Verification items for the finished model (mm, model axes). A direction names the side the tool comes from. Coordinates: 2 decimals unless noted, no trailing zeros. Loops run counter-clockwise (first coordinate to the right, second up) from the corner with the lowest first, then second, coordinate; pieces in that order, holes last. Notation, with made-up numbers: (72.25, 19) -> (100.25, 19) arc R11 cw to (100.25, 31) -> close; hole circle Ø5 at (-35, 69.5). An arc over 180 degrees is marked (long way). Answer as a JSON object with one key per item and string values. Group by question number.
Q1. Release check for a two-part mould opening along Y. For faces 5 (the cylindrical face through (1467.341, 1019.425, 1.815)), 6 (the flat face through (0, -1, -1)), 7 (the flat face through (3.175, -1, -1)) record: released by +Y, released by -Y, zero draft, split by the parting line, or undercut.
Q2. Cross-section at A-A on x = 208.5. Record the boundary of the cut face in (y, z) (3 decimals).
Q3. Set-up check for faces 1 (the cylindrical face through (1467.341, 1095.855, -14.593)), 2 (the flat face through (1510.66, 1097, 12)), 3 (the cylindrical face through (122.164, -30.235, -23.183)), 4 (the cylindrical face through (120.599, -8.948, -40.293)): record each of +Z, -Z, +X, -X, +Y, -Y from which the full face is reachable in a straight line by a thin tool's end or side.
Q4. Scan lines: L1, parallel to Z at x = 119, y = 0 (3 decimals); L2, parallel to Y at x = 1470, z = 0; L3, parallel to Y at x = 226.5, z = 0.5. Record each from-to range of solid material in increasing order.
Q5. Gauge pin test, flat ends, axial feed: pin 1 Ø12 at (x, z) = (679, 32) entering from -Y; pin 2 Ø10 at (x, z) = (338, 26.5) entering from -Y; pin 3 Ø12 at (x, z) = (1034, -30.5) entering from -Y. Record the tip position at first contact, or that the pin passes through.
```python
from build123d import *

# Parameters (mm, degrees)
BARRER2_PROFILE_R = 41.275
VACIADO1_T        = -3.175


with BuildPart() as part:
    # Barrer2: sweep along a path in Croquis1
    with BuildLine(Plane.XY) as barrer2_path:
        Line((0, 0), (237.867965644, 0))
        ThreePointArc((237.867965644, 0), (295.270480499, 11.418070123), (343.933982822, 43.933982822))
        Line((343.933982822, 43.933982822), (1316.726188958, 1016.726188958))
        ThreePointArc((1316.726188958, 1016.726188958), (1365.389691281, 1049.242101657), (1422.792206136, 1060.66017178))
        Line((1422.792206136, 1060.66017178), (1510.66017178, 1060.66017178))
    # Barrer2 profile (on start of the path) → Barrer2 (sweep)
    with BuildSketch(Plane.YZ):
        Circle(BARRER2_PROFILE_R)
    sweep(path=barrer2_path.line)

    # Vaciado1
    vaciado1_openings = [part.faces().sort_by_distance(p)[0] for p in [
        (1510.66017178, 1060.66017178, 0),
    ]]
    offset(amount=VACIADO1_T, openings=vaciado1_openings, kind=Kind.INTERSECTION)


solid = part.part
```
Computed values:
{
 "1": {"face 5": "split by the parting line", "face 6": "zero draft", "face 7": "undercut"},
 "2": {"outline": "circle Ø82.55 at (0, 0); hole circle Ø76.2 at (0, 0)"},
 "3": {"face 1": "+X", "face 2": "+Z, -Z, +X, +Y, -Y", "face 3": "none", "face 4": "-X"},
 "4": {"L1": "z = -41.275 to -38.1, 38.1 to 41.275", "L2": "y = 1019.39 to 1022.56, 1098.76 to 1101.94", "L3": "y = -41.27 to -38.1, 38.1 to 41.27"},
 "5": {"pin 1": "stops at y = 331.49", "pin 2": "stops at y = -6.99", "pin 3": "stops at y = 684.7"}
}
